Source: three-view drawing plus pictorial views. Frame: mm from the lowest corner of the part. A direction names the side the tool comes from. Round coordinates to 2 decimals unless told otherwise and drop trailing zeros. Order: outer loops, then holes, each group sorted by start corner. A loop starts at its lowest first (then second) coordinate and runs counter-clockwise, first axis right, second up. Notation, with made-up numbers: (-15.75, 37) - (1.25, 37) arc R28 ccw to (1.25, 74) - close; hole circle Ø9 at (-30.5, -15). An arc over 180 degrees is marked (long way). One line per item, written item: value. Start each with the question number.
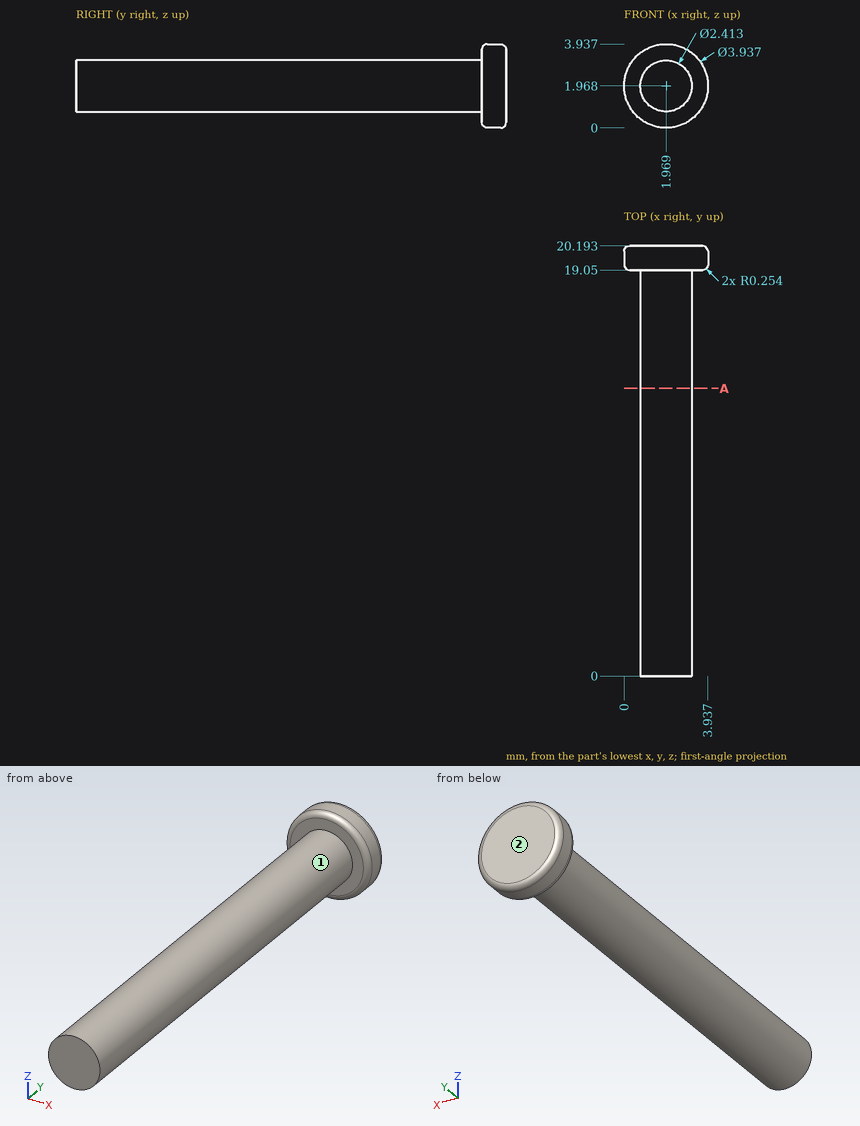
Item 1: Line query: L1, parallel to Y at x = 2.05, z = 3.45; L2, parallel to Z at x = 1.95, y = 17 (1 decimal); L3, parallel to X at y = 15.75, z = 1.6. Output: solid intervals per line, ascending.
Item 2: First-contact query: pin 1 Ø1.5 at (x, y) = (1, 4.5) entering from +Z (1 decimal); pin 2 Ø1 at (y, z) = (16.5, 0.5) entering from +X. Flat tips, straight axial feed; report the tip coordinate or a pass-through.
Item 3: Reachability of the marked faces 1 and 2 from +Z, -Z, +X, -X, +Y, -Y: full face, straight path, thin tool, end or side. Return the list, or none.
Item 4: Section query A-A on y = 13.5. Return loops of the section in (x, z).
Geometry results:
1. L1: y = 19.05 to 20.19
1. L2: z = 0.8 to 3.2
1. L3: x = 0.82 to 3.12
2. pin 1: stops at z = 3.2
2. pin 2: stops at x = 2.69
3. face 1: -Y
3. face 2: +Z, -Z, +X, -X, +Y
4. outline: circle Ø2.41 at (1.97, 1.97)
